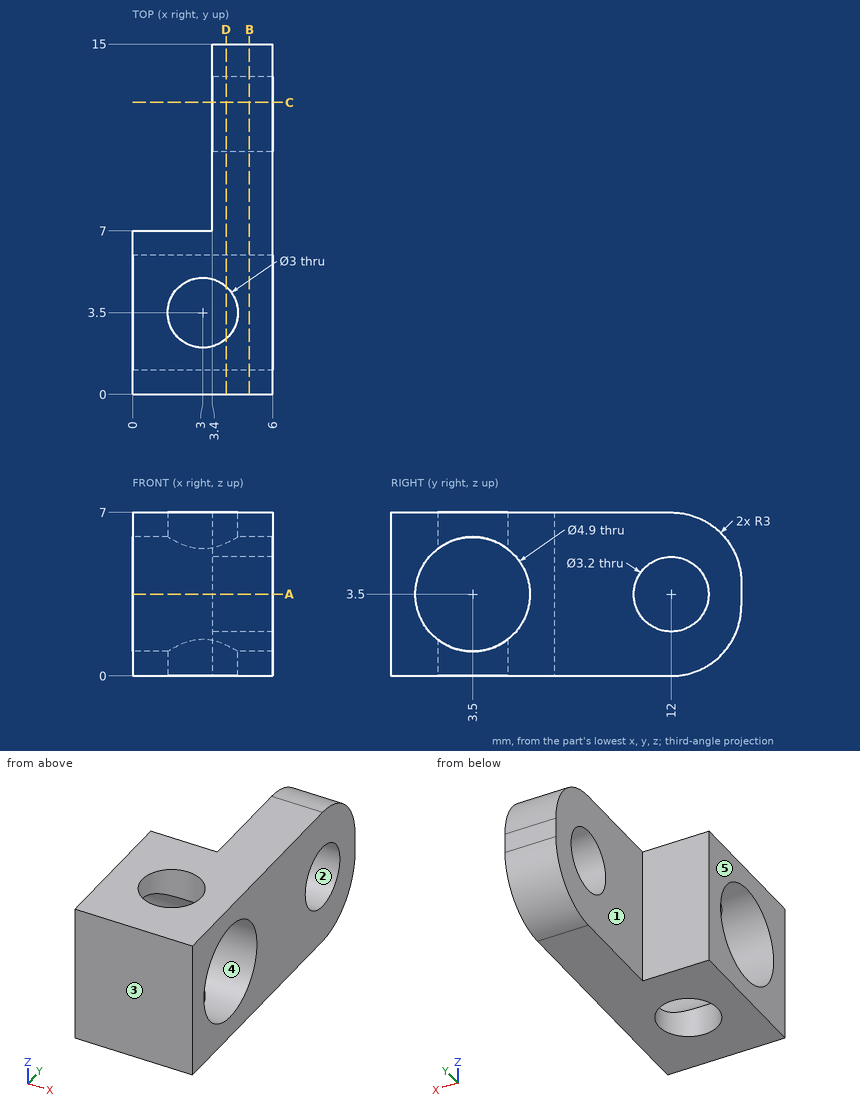
Check sheet for the drawn part. Datum: minimum x, y, z corner. Units: mm. A direction names the side the tool comes from. Coordinates: 2 decimals unless noted, no trailing zeros. Write each loop counter-clockwise with the first axis right and the second up, starting at its lowest first coordinate (ties: lowest second). Pieces come first, ordered by that corner, then holes. Notation, with made-up numbers: (-15, 75) - (14, 75) arc R17 cw to (14, 88) - close; hole circle Ø11 at (0.25, -38). An arc over 180 degrees is marked (long way). Answer as a JSON object with one key per item and string values.
(1) Thickness scan on line 1 along Y through (x, z) = (3, 5.85); line 2 along X through (y, z) = (3.5, 6.6); line 3 along Z through (x, y) = (4.7, 12). Record the ranges inside material, lowest first.
Report:
{"line 1": "0 to 2, 5 to 7", "line 2": "0 to 1.5, 4.5 to 6", "line 3": "0 to 1.9, 5.1 to 7"}
(2) Cross-section at A-A on z = 3.5. Record the cut outline in (x, y).
Report:
{"outline": "(0, 0) - (6, 0) - (6, 1.05) - (0, 1.05) - close; (0, 5.95) - (6, 5.95) - (6, 10.4) - (3.4, 10.4) - (3.4, 7) - (0, 7) - close; (3.4, 13.6) - (6, 13.6) - (6, 15) - (3.4, 15) - close"}
(3) Gauge pin test, flat end, axial feed: pin 1 Ø1 at (x, z) = (0.5, 4.5) entering from -Y. Record the tip position at first contact, or that the pin passes through.
Report:
{"pin 1": "y = 0"}
(4) Cross-section at C-C on y = 12.5. Record the cut outline in (x, z).
Report:
{"outline": "(3.4, 0.04) - (6, 0.04) - (6, 1.98) - (3.4, 1.98) - close; (3.4, 5.02) - (6, 5.02) - (6, 6.96) - (3.4, 6.96) - close"}
(5) Tool access check on the marked faces 1 and 2. Record the directions out of +Z, -Z, +X, -X, +Y, -Y that give a thin tool (end or side, any length) a straight path to the whole face; none if there is none.
Report:
{"face 1": "+Z, -Z, -X, +Y", "face 2": "+X, -X"}
(6) Cross-section at D-D on x = 4. Record the cut outline in (y, z).
Report:
{"outline": "(0, 0) - (2.38, 0) - (2.38, 1.32) arc R2.45 cw to (2.38, 5.68) - (2.38, 7) - (0, 7) - close; (4.62, 0) - (12, 0) arc R3 ccw to (15, 3) - (15, 4) arc R3 ccw to (12, 7) - (4.62, 7) - (4.62, 5.68) arc R2.45 cw to (4.62, 1.32) - close; hole circle Ø3.2 at (12, 3.5)"}
(7) Mould release check, pull along Y, two halves, no side actions. Record for the marked faces 3, 4 and 5: pulls with the +Y half, pulls with the -Y half, needs draft (parallel to the pull), parting line crosses it, or undercut.
Report:
{"face 3": "pulls with the -Y half", "face 4": "undercut", "face 5": "needs draft"}
(8) Cross-section at B-B on x = 5. Record the cut outline in (y, z), plus the area to 3 significant figures.
Report:
{"outline": "(0, 0) - (12, 0) arc R3 ccw to (15, 3) - (15, 4) arc R3 ccw to (12, 7) - (0, 7) - close; hole circle Ø4.9 at (3.5, 3.5); hole circle Ø3.2 at (12, 3.5)", "area": "74.2 mm^2"}
